Verification items for the finished model (mm, model axes). A direction names the side the tool comes from. Coordinates: 2 decimals unless noted, no trailing zeros. Loops run counter-clockwise (first coordinate to the right, second up) from the corner with the lowest first, then second, coordinate; pieces in that order, holes last. Notation, with made-up numbers: (7, 4) - (23, 4) arc R10 cw to (23, 12) - close; hole circle Ø10 at (64.25, -28). An arc over 180 degrees is marked (long way). One line per item, written item: value. Start each with the question number.
(1) Section check B-B (z = 8). Record the boundary of the cut face in (x, y), plus the area to 3 significant figures.
(2) Draft check along X on faces 3 (the face through (3.045, 1.726, 4.986)), 4 (the face through (1, 3, 4)), 5 (the face through (-0.14, 0.63, 2.81)). Enter one of: +X half, -X half, draft (parallel to the pull), parting line (faces both ways), or undercut.
(3) Thickness scan on probe 1 along Y at (x, z) = (0, 7.95); probe 2 along X at (y, z) = (0.5, 8); probe 3 along X at (y, z) = (-0.25, 0.75). Record the ranges inside material, lowest first. Write a range as [from, to].
(4) Section check A-A (x = 0). Record the boundary of the cut face in (y, z).
(5) Gauge pin test, flat ends, axial feed: P1, Ø2.5, axis at x = 0, y = 0, coming from the +Z side; P2, Ø1.5, axis at x = 1, z = 3, coming from the +Y side; P3, Ø2, axis at y = 2, z = 6, coming from the +X side; P4, Ø3, axis at y = -1.5, z = 2, coming from the +X side. Record the tip position at first contact, or that the pin passes through.
(6) Set-up check for faces 1 (the face through (-1, 3, 6)), 2 (the face through (-3.045, -1.726, 4.986)): record each of +Z, -Z, +X, -X, +Y, -Y from which the full face is reachable in a straight line by a thin tool's end or side.
```python
from build123d import *

# Parameters (mm, degrees)
BOSS_EXTRU_1_DEPTH      = 9
ESQUISSE2_W             = 19.623971562
ESQUISSE2_H             = 15.534154535
ESQUISSE2_R             = 3
ENL_V_MAT_EXTRU_1_DEPTH = 3
ENL_V_START             = -4
ESQUISSE3_W             = 11.267201257
ESQUISSE3_H             = 13.961169169
ESQUISSE3_R             = 3
ENL_V_MAT_EXTRU_2_DEPTH = 4
CHANFREIN1_SIZE         = 4
CHANFREIN1_SIZE_2       = 2.499477408


with BuildPart() as part:
    # Esquisse1 → Boss.-Extru.1 (new body)
    with BuildSketch(Plane.XY):
        Polygon((4.041451884, 0), (2.020725942, 3.5), (-2.020725942, 3.5), (-4.041451884, 0), (-2.020725942, -3.5), (2.020725942, -3.5), align=None)
    extrude(amount=BOSS_EXTRU_1_DEPTH)

    # Esquisse2 → Enlèv. mat.-Extru.1 (cut)
    with BuildSketch(Plane.XY.offset(9)):
        with Locations((0.327116653, -1.544441398)):
            Rectangle(ESQUISSE2_W, ESQUISSE2_H)
        Circle(ESQUISSE2_R, mode=Mode.SUBTRACT)
    extrude(amount=-ENL_V_MAT_EXTRU_1_DEPTH, mode=Mode.SUBTRACT)

    # Esquisse3 → Enlèv. mat.-Extru.2 (cut)
    with BuildSketch(Plane(origin=(0, 0, 0), x_dir=(-1, 0, 0), z_dir=(0, 0, -1)).offset(ENL_V_START)):
        with Locations((0.009770186, 0.039262349)):
            Rectangle(ESQUISSE3_W, ESQUISSE3_H)
        with Locations(Location((0, 0, 0), (0, 0, 180))):
            Circle(ESQUISSE3_R, mode=Mode.SUBTRACT)
    extrude(amount=ENL_V_MAT_EXTRU_2_DEPTH, mode=Mode.SUBTRACT)

    # Chanfrein1
    # the kernel refuses this chamfer: 4, 2.499477408 mm, written as the material it takes off along each edge
    with BuildSketch(Plane(origin=(0, 0, 0), x_dir=(1, 0, 0), z_dir=(0, 1, 0))) as chanfrein1_piece_1_section:
        Polygon((3, -CHANFREIN1_SIZE), (3 - CHANFREIN1_SIZE_2, 0), (3, 0), align=None)
    chanfrein1_piece_1 = revolve(axis=Axis((0, 0, 0), (0, 0, -1)), mode=Mode.PRIVATE)
    chanfrein1_piece_1 = split(chanfrein1_piece_1, bisect_by=Plane(origin=(-1.744026904, 0, 4), z_dir=(0, 0, -1)), keep=Keep.TOP, mode=Mode.PRIVATE)
    add(chanfrein1_piece_1, mode=Mode.SUBTRACT)

    # Esquisse4 → Enlèvement de matière-Révolution1 (revolve, cut)
    with BuildSketch(Plane(origin=(0, 0, 0), x_dir=(1, 0, 0), z_dir=(0, 1, 0))):
        Polygon((0, -9), (1, -9), (1, -5.7010425), (0.3, 0), (0, 0), align=None)
    revolve(axis=Axis((0, 0, 10.381605157), (0, 0, -1)), mode=Mode.SUBTRACT)


solid = part.part
```
Responses:
1. outline: circle Ø6 at (0, 0); hole circle Ø2 at (0, 0)
1. area: 25.1 mm²
2. face 3: +X half
2. face 4: draft
2. face 5: undercut
3. probe 1: y = [-3, -1], [1, 3]
3. probe 2: x = [-2.96, -0.87], [0.87, 2.96]
3. probe 3: x = [-0.94, -0.3], [0.3, 0.94]
4. outline: (-3.5, 4) - (-3, 4) - (-0.5, 0) - (-0.3, 0) - (-1, 5.7) - (-1, 9) - (-3, 9) - (-3, 6) - (-3.5, 6) - close; (0.3, 0) - (0.5, 0) - (3, 4) - (3.5, 4) - (3.5, 6) - (3, 6) - (3, 9) - (1, 9) - (1, 5.7) - close
5. P1: stops at z = 9
5. P2: stops at y = 2.72
5. P3: stops at x = 3.46
5. P4: stops at x = 2.45
6. face 1: +Z
6. face 2: +Z, -Z, -X, -Y
